Autodesk Inventor part; units mm, degrees
ref_plane "YZ Plane" through (0, 0, 0) normal (1, 0, 0) x (0, 1, 0)
ref_plane "XZ Plane" through (0, 0, 0) normal (0, 1, 0) x (-1, 0, 0)
ref_plane "XY Plane" through (0, 0, 0) normal (0, 0, 1) x (1, 0, 0)
sketch "Sketch1" plane through (0, 0, 0) normal (0, 0, 1) x (1, 0, 0)
  circle A0 centre (167.1084, 53.7786) radius 29.5
  line L0 (167.1084, 83.2786) -> (115.1084, 83.2786)
  line L1 (115.1084, 83.2786) -> (115.1084, 24.2786)
  line L2 (115.1084, 24.2786) -> (167.1084, 24.2786)
  circle A1 centre (167.1084, 53.7786) radius 9.525
  circle A2 centre (145.2715, 55.689) radius 2
  circle A3 centre (169.0189, 75.6154) radius 2
  circle A4 centre (188.9453, 51.8681) radius 2
  circle A5 centre (165.1979, 31.9417) radius 2
  line L3 (169.0189, 75.6154) -> (165.1979, 31.9417) construction
  line L4 (188.9453, 51.8681) -> (145.2715, 55.689) construction
  line L5 (-39.3217, 0) -> (235.9301, 0)
  line L6 (0, -16.6557) -> (0, 99.9343)
  line L7 (167.1084, 53.7786) -> (100.0684, 53.7786) construction
  circle A6 centre (122.0877, 71.2786) radius 2.0193
  circle A7 centre (127.0877, 71.2786) radius 2.0193
  circle A8 centre (137.0877, 71.2786) radius 2.0193
  circle A9 centre (142.0877, 71.2786) radius 2.0193
  circle A10 centre (127.0877, 36.2786) radius 2.0193
  circle A11 centre (122.0877, 36.2786) radius 2.0193
  circle A12 centre (142.0877, 36.2786) radius 2.0193
  circle A13 centre (137.0877, 36.2786) radius 2.0193
  line L8 (127.0877, 73.2979) -> (122.0877, 73.2979)
  line L9 (122.0877, 69.2593) -> (127.0877, 69.2593)
  line L10 (137.0877, 73.2979) -> (142.0877, 73.2979)
  line L11 (142.0877, 69.2593) -> (137.0877, 69.2593)
  line L12 (142.0877, 38.2979) -> (137.0877, 38.2979)
  line L13 (137.0877, 34.2593) -> (142.0877, 34.2593)
  line L14 (127.0877, 38.2979) -> (122.0877, 38.2979)
  line L15 (122.0877, 34.2593) -> (127.0877, 34.2593)
  circle A14 centre (125.0684, 71.2786) radius 2.0193 construction
  circle A15 centre (125.0684, 36.2786) radius 2.0193 construction
  line L16 (125.0684, 71.2786) -> (125.0684, 36.2786) construction
  circle A16 centre (140.0684, 36.2786) radius 2.0193 construction
  circle A17 centre (140.0684, 71.2786) radius 2.0193 construction
  line L17 (140.0684, 71.2786) -> (140.0684, 36.2786) construction
  point P0 (0, 0)
  dimension "d0" = 59
  dimension "d1" = 52
  dimension "d2" = 19.05
  dimension "d3" = 4
  dimension "d4" = 4
  dimension "d5" = 4
  dimension "d6" = 4
  dimension "d7" = 355
  dimension "d8" = 31
  dimension "d9" = 31
  dimension "d10" = 31
  dimension "d11" = 67.04
  dimension "d13" = 4.0386
  dimension "d14" = 4.0386
  dimension "d16" = 4.0386
  dimension "d17" = 4.0386
  dimension "d18" = 4.0386
  dimension "d19" = 4.0386
  dimension "d20" = 4.0386
  dimension "d21" = 4.0386
  dimension "d22" = 5
  dimension "d23" = 5
  dimension "d24" = 5
  dimension "d25" = 5
  dimension "d26" = 4.0386
  dimension "d27" = 25
  dimension "d29" = 15
  dimension "d32" = 35
extrude "Extrusion1" add sketch "Sketch1" along normal blind 3.175 contours A0 A12 A9 | A0 A9 L10 A8 L11 L12 A13 L13 A12 L2 L1 L0
properties part number "MMplate2"
The model under review builds one solid part; all positions refer to its coordinate system, in mm. A direction names the side the tool comes from. Coordinates: 2 decimals unless noted, no trailing zeros. Write each loop counter-clockwise with the first axis right and the second up, starting at its lowest first coordinate (ties: lowest second). Pieces come first, ordered by that corner, then holes. Notation, with made-up numbers: (70.25, 43.5) -> (121.25, 43.5) arc R22 ccw to (121.25, 58.5) -> close; hole circle Ø8 at (80.25, 60). An arc over 180 degrees is marked (long way). One line per item, written item: value. Start each with the question number.
Q1. Clearance check with flat-ended pins moving along their axes: P1, Ø4.5, axis at x = 188.95, y = 51.87, coming from the -Z side; P2, Ø1, axis at y = 76, z = 2, coming from the +X side. State where each tip first meets the part, or that it passes through.
Q2. For faces 4 (the face through (141, 24.279, 2)), 5 (the face through (140, 38.298, 2)), list the 3-axis set-ups (+Z, -Z, +X, -X, +Y, -Y) from which the entire face can be reached by the end or side of a thin tool; tool diameter is ignored.
Q3. Add section A-A, the plane x = 162. Give the boundary of the cut face in (y, z) (3 decimals).
Q4. Add section C-C, the plane y = 49. Give the boundary of the cut face in (x, z) (3 decimals), then the cut area to 3 significant figures.
Q5. The part is to be moulded in two halves that separate along Y. For faces 1 (the face through (141, 83.279, 2)), 2 (the face through (115.108, 54, 2)), 3 (the face through (140, 69.259, 2)), say which applies: +Y half, -Y half, draft (parallel to the pull), parting line (faces both ways), or undercut.
Q6. To check wall thickness, follow probe 1 along Y at (x, z) = (137.5, 2.75); probe 2 along Y at (x, z) = (169.5, 0.75); probe 3 along X at (y, z) = (34.5, 3.05). State the ranges of each line that lie inside material, in increasing order.
Q7. Add section B-B, the plane z = 1.8. Count the separate pieces of the cut face and the enclosed holes in it, then the cut area to 3 significant figures.
Q8. Add section D-D, the plane x = 185. Give the boundary of the cut face in (y, z) (3 decimals).
Response:
1. P1: z = 0
1. P2: x = 187.07
2. face 4: +Z, -Z, +X, -X, -Y
2. face 5: +Z, -Z
3. outline: (24.279, 0) -> (45.739, 0) -> (45.739, 3.175) -> (24.279, 3.175) -> close; (61.818, 0) -> (83.279, 0) -> (83.279, 3.175) -> (61.818, 3.175) -> close
4. outline: (115.108, 0) -> (158.869, 0) -> (158.869, 3.175) -> (115.108, 3.175) -> close; (175.348, 0) -> (196.219, 0) -> (196.219, 3.175) -> (175.348, 3.175) -> close
4. area: 205 mm²
5. face 1: +Y half
5. face 2: draft
5. face 3: undercut
6. probe 1: 24.28 to 34.26, 38.3 to 69.26, 73.3 to 83.28
6. probe 2: 24.38 to 44.56, 63 to 73.67, 77.56 to 83.18
6. probe 3: 115.11 to 121.13, 128.04 to 136.13, 143.04 to 189.44
7. separate pieces: 1
7. enclosed holes: 9
7. area: 3,970 mm²
8. outline: (30.324, 0) -> (77.234, 0) -> (77.234, 3.175) -> (30.324, 3.175) -> close
